Here's the drawing with two shaded views (mm, measured from the low corner). I have some questions. A direction names the side the tool comes from. Give positions to 0.01 mm unless a question says otherwise; leave off trailing zeros. Loops run counter-clockwise (first coordinate to the right, second up) from the corner with the lowest first, then second, coordinate; pieces in that order, holes last. Notation, with made-up numbers: (19.25, 48.25) -> (58.25, 48.25) arc R21 cw to (58.25, 58.25) -> close; hole circle Ø6 at (51, 55.5). An arc over 180 degrees is marked (long way). Put each result on its own line as item: value.
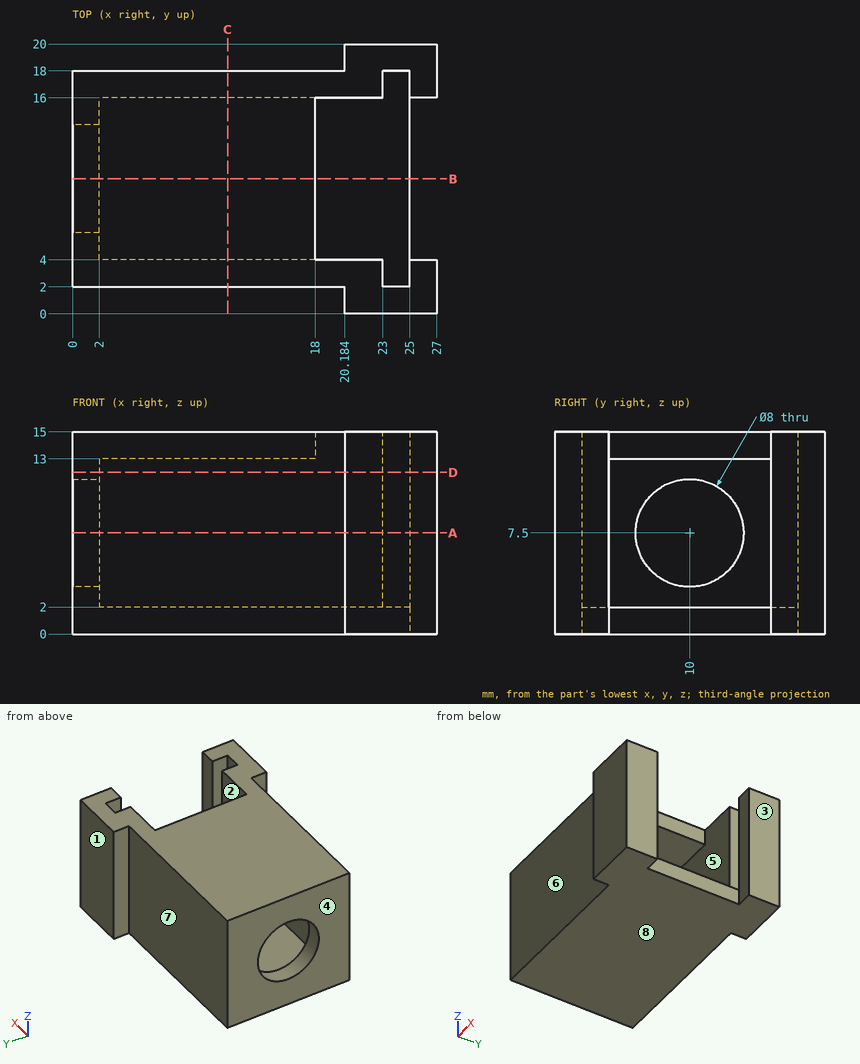
1. If we section it at C-C (x = 11.5): List the corners of the cut face in (y, z) for me.
Recorded:
outline: (2, 0) -> (18, 0) -> (18, 15) -> (2, 15) -> close; hole (4, 2) -> (16, 2) -> (16, 13) -> (4, 13) -> close
2. If we section it at B-B (y = 10): List the corners of the cut face in (x, z) for me, then the cut area to 3 significant figures.
Recorded:
outline: (0, 0) -> (25, 0) -> (25, 2) -> (2, 2) -> (2, 3.5) -> (0, 3.5) -> close; (0, 11.5) -> (2, 11.5) -> (2, 13) -> (18, 13) -> (18, 15) -> (0, 15) -> close
area: 92.0 mm^2
3. I need wall thicknesses on line 1 (Z direction, x = 16.5, y = 13); line 2 (Y direction, x = 1.2, z = 7.5); line 3 (Y direction, x = 15, z = 5). Which ranges of each line are inside material? Lowest first, please.
Recorded:
line 1: z = 0 to 2, 13 to 15
line 2: y = 2 to 6, 14 to 18
line 3: y = 2 to 4, 16 to 18
4. Thinking about a two-plate mould opening in Y: for the marked faces 1, 2 and 3, which applies, pulls with the +Y half, pulls with the -Y half, needs draft (parallel to the pull), parting line crosses it, or undercut?
Recorded:
face 1: pulls with the +Y half
face 2: undercut
face 3: needs draft
5. For the marked faces 4, 5, 6, 7 and 8, which set-ups out of +Z, -Z, +X, -X, +Y, -Y let a thin tool reach every point of the face, with its end or its side?
Recorded:
face 4: +Z, -Z, -X, +Y, -Y
face 5: +X
face 6: +Z, -Z, -X, -Y
face 7: +Z, -Z, -X, +Y
face 8: -Z, +X, -X, +Y, -Y
6. If we section it at D-D (z = 12): List the corners of the cut face in (x, y) for me, then the cut area to 3 significant figures.
Recorded:
outline: (0, 2) -> (20.18, 2) -> (20.18, 0) -> (27, 0) -> (27, 4) -> (25, 4) -> (25, 2) -> (23, 2) -> (23, 4) -> (2, 4) -> (2, 16) -> (23, 16) -> (23, 18) -> (25, 18) -> (25, 16) -> (27, 16) -> (27, 20) -> (20.18, 20) -> (20.18, 18) -> (0, 18) -> close
area: 151 mm^2
7. If we section it at A-A (z = 7.5): List the corners of the cut face in (x, y) for me.
Recorded:
outline: (0, 2) -> (20.18, 2) -> (20.18, 0) -> (27, 0) -> (27, 4) -> (25, 4) -> (25, 2) -> (23, 2) -> (23, 4) -> (2, 4) -> (2, 6) -> (0, 6) -> close; (0, 14) -> (2, 14) -> (2, 16) -> (23, 16) -> (23, 18) -> (25, 18) -> (25, 16) -> (27, 16) -> (27, 20) -> (20.18, 20) -> (20.18, 18) -> (0, 18) -> close
8. I'm going to push flat-ended pins straight in: pin 1 (7 mm diameter, centred on y = 10, z = 7.5, fed in from -X); pin 2 (1 mm diameter, centred on x = 24, z = 5.5, fed in from -Y); pin 3 (0.6 mm diameter, centred on y = 18.5, z = 8, fed in from -X); pin 4 (6.5 mm diameter, centred on x = 8, z = 11, fed in from -Y). Where does each tip first touch, or does it pass through?
Recorded:
pin 1: passes through
pin 2: stops at y = 0
pin 3: stops at x = 20.18
pin 4: stops at y = 2
